```python
from build123d import *

# Parameters (mm, degrees)
SKETCH1_W                                            = 76.36
SKETCH1_H                                            = 74
BOSS_EXTRUDE1_DEPTH                                  = 6
FILLET1_R                                            = 2
FILLET2_R                                            = 2
FILLET3_R                                            = 2
FILLET4_R                                            = 2
CSK_FOR_M2_COUNTERSUNK_RAISED_HEAD_SCREW_D           = 2.4
CSK_FOR_M2_COUNTERSUNK_RAISED_HEAD_SCREW_CSINK_D     = 4.4
CSK_FOR_M2_COUNTERSUNK_RAISED_HEAD_SCREW_CSINK_ANGLE = 90
BOSS_EXTRUDE2_DEPTH                                  = 38.3
CUT_EXTRUDE1_DEPTH                                   = 36.3
SKETCH8_W                                            = 37.9
SKETCH8_H                                            = 21.6
CUT_EXTRUDE2_DEPTH                                   = 10


with BuildPart() as part:
    # Sketch1 → Boss-Extrude1 (new body)
    with BuildSketch(Plane.XY):
        with Locations((5.593243707, -7.586756293)):
            Rectangle(SKETCH1_W, SKETCH1_H)
    extrude(amount=BOSS_EXTRUDE1_DEPTH)

    # Fillet1
    fillet1_edges = [part.edges().sort_by_distance(p)[0] for p in [
        (-32.586756293, 29.413243707, 3),
    ]]
    fillet(fillet1_edges, radius=FILLET1_R)

    # Fillet2
    fillet2_edges = [part.edges().sort_by_distance(p)[0] for p in [
        (43.773243707, 29.413243707, 3),
    ]]
    fillet(fillet2_edges, radius=FILLET2_R)

    # Fillet3
    fillet3_edges = [part.edges().sort_by_distance(p)[0] for p in [
        (-32.586756293, -44.586756293, 3),
    ]]
    fillet(fillet3_edges, radius=FILLET3_R)

    # Fillet4
    fillet4_edges = [part.edges().sort_by_distance(p)[0] for p in [
        (43.773243707, -44.586756293, 3),
    ]]
    fillet(fillet4_edges, radius=FILLET4_R)

    # CSK for M2 Countersunk Raised Head Screw1 (through all)
    with Locations(Plane.XY.offset(6)):
        with Locations((-26.066697121, 22.893243707), (37.255416012, -38.066697121)):
            CounterSinkHole(CSK_FOR_M2_COUNTERSUNK_RAISED_HEAD_SCREW_D / 2, CSK_FOR_M2_COUNTERSUNK_RAISED_HEAD_SCREW_CSINK_D / 2, counter_sink_angle=CSK_FOR_M2_COUNTERSUNK_RAISED_HEAD_SCREW_CSINK_ANGLE)

    # Sketch2 → Boss-Extrude2 (add)
    with BuildSketch(Plane.XY):
        Polygon((42.073243707, -26.488928598), (42.073243707, 27.673243707), (-14.526756293, 27.673243707), (-30.886756293, 11.313243707), (-30.886756293, -42.886756293), (25.675416012, -42.886756293), align=None)
    extrude(amount=BOSS_EXTRUDE2_DEPTH)

    # Sketch3 → Cut-Extrude1 (cut)
    with BuildSketch(Plane(origin=(0, 0, 0), x_dir=(-1, 0, 0), z_dir=(0, 0, -1))):
        Polygon((-25.168605052, -40.786756293), (28.786756293, -40.786756293), (28.786756293, 10.491732857), (13.386650304, 25.613243707), (-39.791667004, 25.613243707), (-39.975416012, -26.119028061), align=None)
    extrude(amount=-CUT_EXTRUDE1_DEPTH, mode=Mode.SUBTRACT)

    # Sketch8 → Cut-Extrude2 (cut)
    with BuildSketch(Plane.XZ.offset(42.886756293)):
        with Locations((-6, 22)):
            Rectangle(SKETCH8_W, SKETCH8_H)
    extrude(amount=-CUT_EXTRUDE2_DEPTH, mode=Mode.SUBTRACT)


solid = part.part
```
Check sheet for the modelled part. Datum: model origin and axes. Units: mm. A direction names the side the tool comes from. Round coordinates to 2 decimals unless told otherwise and drop trailing zeros. Order: outer loops, then holes, each group sorted by start corner. A loop starts at its lowest first (then second) coordinate and runs counter-clockwise, first axis right, second up. Notation, with made-up numbers: (16, 35) -> (62, 35) arc R22 ccw to (62, 56) -> close; hole circle Ø9 at (-5.5, 28.5). An arc over 180 degrees is marked (long way). One line per item, written item: value. Start each with the question number.
Q1. Cross-section at A-A (x = -2). Record the boundary of the cut face in (y, z).
Q2. Cross-section at B-B (z = 9). Record the boundary of the cut face in (x, y), and give its area (3 significant figures).
Q3. Mould release check, pull along Y, two halves, no side actions. Record for faces 4 (the face through (-32.587, -8, 3)), 5 (the face through (-1, -40.787, 10)), 6 (the face through (33.76, -34.8, 21.92)): pulls with the +Y half, pulls with the -Y half, needs draft (parallel to the pull), parting line crosses it, or undercut.
Q4. Cross-section at D-D (y = 2). Record the boundary of the cut face in (x, z), and give its area (3 significant figures).
Q5. Gauge pin test, flat ends, axial feed: pin 1 Ø16 at (y, z) = (10.5, 15) entering from +X; pin 2 Ø11 at (x, z) = (6, 18.5) entering from -Y; pin 3 Ø12 at (x, z) = (-9, 20) entering from +Y. Record the tip position at first contact, or that the pin passes through.
Q6. Cross-section at C-C (x = 17). Record the boundary of the cut face in (y, z).
Q7. Thickness scan on line 1 (Y direction, x = 9, z = 34); line 2 (Y direction, x = -3, z = 2); line 3 (X direction, y = -22, z = 29.5). Record the ranges inside material, lowest first.
Q8. Set-up check for faces 1 (the face through (-24.95, -42, 22)), 2 (the face through (-21.19, 17.95, 17.9)), 3 (the face through (14, 27.673, 22)): record each of +Z, -Z, +X, -X, +Y, -Y from which the full face is reachable in a straight line by a thin tool's end or side.
Completed:
1. outline: (-44.59, 0) -> (-40.79, 0) -> (-40.79, 11.2) -> (-42.89, 11.2) -> (-42.89, 6) -> (-44.59, 6) -> close; (-42.89, 32.8) -> (-40.79, 32.8) -> (-40.79, 36.3) -> (25.61, 36.3) -> (25.61, 0) -> (29.41, 0) -> (29.41, 6) -> (27.67, 6) -> (27.67, 38.3) -> (-42.89, 38.3) -> close
2. outline: (-30.89, -42.89) -> (25.68, -42.89) -> (42.07, -26.49) -> (42.07, 27.67) -> (-14.53, 27.67) -> (-30.89, 11.31) -> close; hole (-28.79, -40.79) -> (25.17, -40.79) -> (39.98, -26.12) -> (39.79, 25.61) -> (-13.39, 25.61) -> (-28.79, 10.49) -> close
2. area: 544 mm²
3. face 4: needs draft
3. face 5: undercut
3. face 6: pulls with the -Y half
4. outline: (-32.59, 0) -> (-28.79, 0) -> (-28.79, 36.3) -> (39.88, 36.3) -> (39.88, 0) -> (43.77, 0) -> (43.77, 6) -> (42.07, 6) -> (42.07, 38.3) -> (-30.89, 38.3) -> (-30.89, 6) -> (-32.59, 6) -> close
4. area: 322 mm²
5. pin 1: stops at x = 42.07
5. pin 2: stops at y = 25.61
5. pin 3: stops at y = 27.67
6. outline: (-44.59, 0) -> (-40.79, 0) -> (-40.79, 36.3) -> (25.61, 36.3) -> (25.61, 0) -> (29.41, 0) -> (29.41, 6) -> (27.67, 6) -> (27.67, 38.3) -> (-42.89, 38.3) -> (-42.89, 6) -> (-44.59, 6) -> close
7. line 1: y = -42.89 to -40.79, 25.61 to 27.67
7. line 2: y = -44.59 to -40.79, 25.61 to 29.41
7. line 3: x = -30.89 to -28.79, 39.96 to 42.07
8. face 1: -Y
8. face 2: -Z
8. face 3: +Z, +X, -X, +Y
